from build123d import *

# Parameters (mm, degrees)
SKIZZE3_W                       = 5
SKIZZE3_H                       = 23
SCHNITT_LINEAR_AUSTRAGEN1_DEPTH = 9
FASE1_SIZE                      = 0.5


with BuildPart() as part:
    # Skizze2 → Rotation1 (revolve)
    with BuildSketch(Plane(origin=(0, 0, 0), x_dir=(0, 0, -1), z_dir=(1, 0, 0)), mode=Mode.PRIVATE) as rotation1_sk:
        Polygon((3, 38), (3, -38), (9.5, -38), (9.5, 21.5), (10, 22), (10, 26), (6, 30), (5, 30), (5, 37.2), (4.2, 38), align=None)
    revolve(rotation1_sk.sketch.rotate(Axis((0, 40.422682589, 0), (0, -1, 0)), 180), axis=Axis((0, 40.422682589, 0), (0, -1, 0)))

    # Skizze3 → Schnitt-Linear austragen1 (cut)
    with BuildSketch(Plane(origin=(0, 30, 0), x_dir=(1, 0, 0), z_dir=(0, 1, 0))):
        with Locations((12, 0)):
            Rectangle(SKIZZE3_W, SKIZZE3_H)
        with Locations((-12, 0)):
            Rectangle(SKIZZE3_W, SKIZZE3_H)
    extrude(amount=-SCHNITT_LINEAR_AUSTRAGEN1_DEPTH, mode=Mode.SUBTRACT)

    # Fase1
    fase1_edges = [part.edges().sort_by_distance(p)[0] for p in [
        (0, 38, -3),
    ]]
    chamfer(fase1_edges, length=FASE1_SIZE)


solid = part.part
Here's how the part is built. I have some questions about the finished solid (model axes, mm). A direction names the side the tool comes from. Round coordinates to 2 decimals unless told otherwise and drop trailing zeros. Order: outer loops, then holes, each group sorted by start corner. A loop starts at its lowest first (then second) coordinate and runs counter-clockwise, first axis right, second up. Notation, with made-up numbers: M -19.5,17 L 27.5,17 A28 cw 27.5,51 Z; hole C -17.75,18 d1. An arc over 180 degrees is marked long. Return JSON: item names as keys, results as strings. Group by question number.
1. If we section it at B-B on y = -25: List the corners of the cut face in (x, z) for me.
2. If we mould it in two halves opening along X, with no side actions, what happens to faces 1 (the face through (-0.9, -0.78, 2.86)), 2 (the face through (-0.21, 21.64, -9.64)), 3 (the face through (-4, 30, -4))? For each: pulls with the +X half, pulls with the -X half, needs draft (parallel to the pull), parting line crosses it, or undercut.
3. On a 3-axis mill with a long thin cutter (end or side, diameter ignored), from which of +Z, -Z, +X, -X, +Y, -Y can I reach the whole of each face in a straight line? I mean faces 4 (the face through (-2.24, -38, 2.24)), 5 (the face through (9.274, -7.834, -2.059)), 6 (the face through (0, 34, -5)). Say none if no direction works.
4. Please list where these lines run through material, in increasing order: probe 1 along X at (y, z) = (17, 0); probe 2 along X at (y, z) = (20, 0.75); probe 3 along X at (y, z) = (15.5, -8.75).
5. If we section it at A-A on x = 0: List the corners of the cut face in (y, z) for me.
6. I'm going to push flat-ended pins straight in: pin 1 Ø2 at (y, z) = (24.5, -4.5) entering from +X; pin 2 Ø3.5 at (x, z) = (-1, 2) entering from +Y; pin 3 Ø5 at (x, y) = (1.5, -15) entering from +Z; pin 4 Ø10 at (x, y) = (7, 3.5) entering from -Z. Where does each tip first touch, or does it pass through?
Reply:
{
 "1": {"outline": "C 0,0 d19; hole C 0,0 d6"},
 "2": {"face 1": "undercut", "face 2": "parting line crosses it", "face 3": "needs draft"},
 "3": {"face 4": "+Z, -Z, +X, -X, -Y", "face 5": "-Y", "face 6": "+Y"},
 "4": {"probe 1": "-9.5 to -3, 3 to 9.5", "probe 2": "-9.47 to -2.9, 2.9 to 9.47", "probe 3": "-3.7 to 3.7"},
 "5": {"outline": "M -38,-9.5 L 21.5,-9.5 L 22,-10 L 26,-10 L 30,-6 L 30,-5 L 37.2,-5 L 38,-4.2 L 38,-3.5 L 37.5,-3 L -38,-3 Z; M -38,3 L 37.5,3 L 38,3.5 L 38,4.2 L 37.2,5 L 30,5 L 30,6 L 26,10 L 22,10 L 21.5,9.5 L -38,9.5 Z"},
 "6": {"pin 1": "x = 9.37", "pin 2": "y = 38", "pin 3": "z = 9.5", "pin 4": "z = -9.29"}
}
